from build123d import *

# Parameters (mm, degrees)
EXTRUDE_1_DEPTH     = 10
SKETCH_2_R          = 1.5
CUT_EXTRUDE_1_DEPTH = 10
SKETCH_3_R          = 1.5
CUT_EXTRUDE_2_DEPTH = 10
SKETCH_5_W          = 49.01
SKETCH_5_H          = 114.02
EXTRUDE_2_DEPTH     = 5
SKETCH_7_W          = 7.579952265
SKETCH_7_H          = 21.325107759
SKETCH_7_H_2        = 11.778124307
SKETCH_7_W_2        = 8.542902392
SKETCH_7_H_3        = 7.419730403
CUT_EXTRUDE_3_DEPTH = 10
SKETCH_8_W          = 6
SKETCH_8_H          = 18.426440066
CUT_EXTRUDE_4_DEPTH = 10
SKETCH_9_R          = 1.5
SKETCH_9_R_2        = 1.621792445
CUT_EXTRUDE_5_DEPTH = 10


with BuildPart() as part:
    # 草图1 → 凸台-拉伸1 (new body)
    with BuildSketch(Plane.XY):
        with BuildLine():
            Line((118, 210), (-118, 210))
            Line((-118, 210), (-118, -210))
            Line((-118, -210), (118, -210))
            Line((118, -210), (118, -50.5))
            Line((118, -50.5), (54.15, -50.5))
            Line((54.15, -50.5), (54.15, -9.334147293))
            ThreePointArc((54.15, -9.334147293), (42.020728949, 0), (54.15, 9.334147293))
            Line((54.15, 9.334147293), (54.15, 50.5))
            Line((54.15, 50.5), (118, 50.5))
            Line((118, 50.5), (118, 210))
        make_face()
    extrude(amount=EXTRUDE_1_DEPTH)

    # 草图2 → 切除-拉伸1 (cut)
    with BuildSketch(Plane.XY.offset(10)):
        with Locations((-88, 135)):
            Circle(SKETCH_2_R)
        with Locations((-43, 180)):
            Circle(SKETCH_2_R)
        with Locations((-88, 180)):
            Circle(SKETCH_2_R)
    extrude(amount=-CUT_EXTRUDE_1_DEPTH, mode=Mode.SUBTRACT)

    # 草图3 → 切除-拉伸2 (cut)
    with BuildSketch(Plane.XY.offset(10)):
        with Locations((51.15, -15.672792958)):
            Circle(SKETCH_3_R)
        with Locations((112.73, -53.5)):
            Circle(SKETCH_3_R)
        with Locations((112.73, -59.5)):
            Circle(SKETCH_3_R)
        with Locations((87.23, -53.5)):
            Circle(SKETCH_3_R)
        with Locations((87.23, -59.5)):
            Circle(SKETCH_3_R)
        with Locations((77.23, -53.5)):
            Circle(SKETCH_3_R)
        with Locations((61.23, -53.5)):
            Circle(SKETCH_3_R)
        with Locations((51.15, -53.5)):
            Circle(SKETCH_3_R)
        with Locations((51.15, -43.5)):
            Circle(SKETCH_3_R)
    cut_extrude_2 = extrude(amount=-CUT_EXTRUDE_2_DEPTH, mode=Mode.SUBTRACT)

    # 镜向1: 切除-拉伸2 across plane
    add(cut_extrude_2.mirror(Plane.ZX), mode=Mode.SUBTRACT)


with BuildPart() as body_2:
    # 草图5 → 凸台-拉伸2 (new body)
    with BuildSketch(Plane.XY.offset(20)):
        with Locations((57.393575669, 0)):
            Rectangle(SKETCH_5_W, SKETCH_5_H)
    extrude(amount=EXTRUDE_2_DEPTH)

    # 草图7 → 切除-拉伸3 (cut)
    with BuildSketch(Plane.XY.offset(25)):
        with Locations((36.372677837, 29.137446121)):
            Rectangle(SKETCH_7_W, SKETCH_7_H)
        with Locations((36.502822244, 5.570937847)):
            Rectangle(SKETCH_7_W, SKETCH_7_H_2)
        with Locations((69.609392324, 53.445086976)):
            Rectangle(SKETCH_7_W_2, SKETCH_7_H_3)
    cut_extrude_3 = extrude(amount=-CUT_EXTRUDE_3_DEPTH, mode=Mode.SUBTRACT)

    # 镜向2: 切除-拉伸3 across plane
    add(cut_extrude_3.mirror(Plane.ZX), mode=Mode.SUBTRACT)

    # 草图8 → 切除-拉伸4 (cut)
    with BuildSketch(Plane.XY.offset(25)):
        with Locations((78.898575669, 18.887565602)):
            Rectangle(SKETCH_8_W, SKETCH_8_H)
    cut_extrude_4 = extrude(amount=-CUT_EXTRUDE_4_DEPTH, mode=Mode.SUBTRACT)

    # 镜向3: 切除-拉伸4 across plane
    add(cut_extrude_4.mirror(Plane.ZX), mode=Mode.SUBTRACT)

    # 草图9 → 切除-拉伸5 (cut)
    with BuildSketch(Plane.XY.offset(25)):
        with Locations((39.158575669, 53.5)):
            Circle(SKETCH_9_R)
        with Locations((62.888575669, 53.5)):
            Circle(SKETCH_9_R)
        with Locations((39.158575669, 43.5)):
            Circle(SKETCH_9_R)
        with Locations((78.88084352, 53.5)):
            Circle(SKETCH_9_R_2)
        with Locations((39.158575669, 15.564892241)):
            Circle(SKETCH_9_R)
        with Locations((78.888575669, 36.510785635)):
            Circle(SKETCH_9_R)
        with Locations((78.888575669, 2.775221774)):
            Circle(SKETCH_9_R)
    cut_extrude_5 = extrude(amount=-CUT_EXTRUDE_5_DEPTH, mode=Mode.SUBTRACT)

    # 镜向5: 切除-拉伸5 across plane
    add(cut_extrude_5.mirror(Plane.ZX), mode=Mode.SUBTRACT)


solid = body_2.part
Can you work these out from the model? Positions are in its coordinate system, mm. A direction names the side the tool comes from. Give positions to 0.01 mm unless a question says otherwise; leave off trailing zeros. Order: outer loops, then holes, each group sorted by start corner. A loop starts at its lowest first (then second) coordinate and runs counter-clockwise, first axis right, second up. Notation, with made-up numbers: M 84,6 L 139,6 A15 cw 139,19 Z; hole C 54,11 d11. An arc over 180 degrees is marked long. One line per item, written item: value.
Item 1: If we section it at D-D on y = -24.5: Write out the boundary of the cut face in (x, z), and give its area (3 significant figures).
Verdict:
outline: M 40.16,20 L 75.9,20 L 75.9,25 L 40.16,25 Z
area: 179 mm2
Item 2: If we mould it in two halves opening along X, with no side actions, what happens to faces 4 (the face through (61.698, -52.587, 22.535)), 5 (the face through (40.163, -29, 23)), 6 (the face through (37, -11.46, 23)), 7 (the face through (40.544, -52.925, 22.535))? For each: pulls with the +X half, pulls with the -X half, needs draft (parallel to the pull), parting line crosses it, or undercut.
Verdict:
face 4: undercut
face 5: pulls with the -X half
face 6: needs draft
face 7: undercut
Item 3: If we section it at C-C on z = 23.8: State how many separate pieces and enclosed holes the cut face has, and give its area (3 significant figures).
Verdict:
separate pieces: 1
enclosed holes: 14
area: 4,660 mm2
Item 4: If we section it at B-B on x = 70.5: Write out the boundary of the cut face in (y, z), and give its area (3 significant figures).
Verdict:
outline: M -49.74,20 L 49.74,20 L 49.74,25 L -49.74,25 Z
area: 497 mm2
Item 5: For faces 1 (the face through (65.338, 53, 23)), 2 (the face through (79, -9.674, 23)), 3 (the face through (36, -39.8, 23)), which set-ups out of +Z, -Z, +X, -X, +Y, -Y let a thin tool reach every point of the face, with its end or its side?
Verdict:
face 1: +Z, -Z, +Y
face 2: +Z, -Z, +X
face 3: +Z, -Z, -X
Item 6: Please list where these lines run through material, in increasing order: line 1 (X direction, y = -53.5, z = 23.5); line 2 (X direction, y = -9.5, z = 22.95); line 3 (X direction, y = 31, z = 21.8).
Verdict:
line 1: 32.89 to 37.66, 40.66 to 61.39, 64.39 to 65.34, 73.88 to 77.26, 80.5 to 81.9
line 2: 40.29 to 81.9
line 3: 40.16 to 81.9
Item 7: For pin 1 (3.5 mm diameter, centred on x = 39.16, y = -53.5, fed in from -Z); pin 2 (2.5 mm diameter, centred on y = 34, z = 23.5, fed in from -X), each with a flat end and sliding along its axis, tell me the tip position at first contact or that it passes through.
Verdict:
pin 1: z = 20
pin 2: x = 40.16
Item 8: If we section it at A-A on y = -43.5: Write out the boundary of the cut face in (x, z), and give its area (3 significant figures).
Verdict:
outline: M 32.89,20 L 37.66,20 L 37.66,25 L 32.89,25 Z; M 40.66,20 L 81.9,20 L 81.9,25 L 40.66,25 Z
area: 230 mm2
